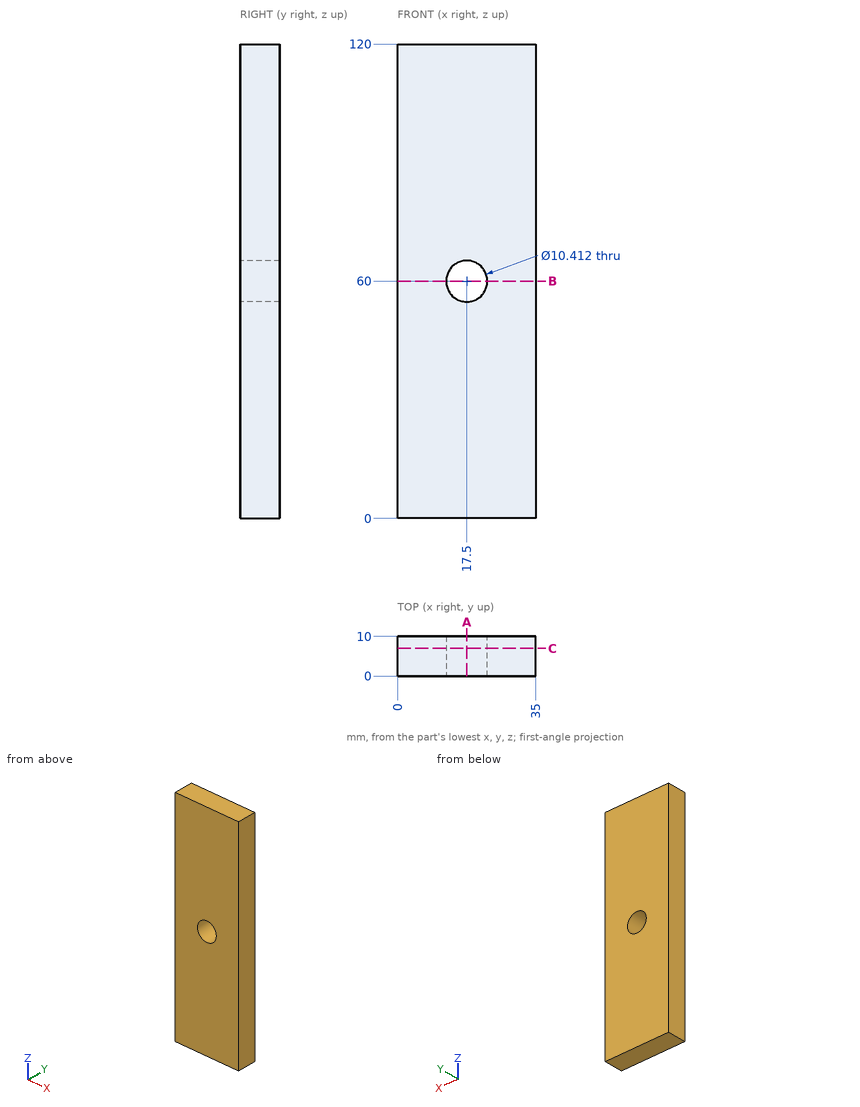
Here's the drawing with two shaded views (mm, measured from the low corner). I have some questions. Give positions to 0.01 mm unless a question says otherwise; leave off trailing zeros. Loops run counter-clockwise (first coordinate to the right, second up) from the corner with the lowest first, then second, coordinate; pieces in that order, holes last. Notation, with made-up numbers: M 0.25,2 L 37.25,2 A27 ccw 37.25,29 Z; hole C 89,24 d3. An arc over 180 degrees is marked long. Use one line per item in the form item = value. Start each with the question number.
Q1. I need wall thicknesses on line 1 along Z through (x, y) = (17.5, 4) (1 decimal); line 2 along X through (y, z) = (8.5, 60.5); line 3 along Z through (x, y) = (16.5, 5.5). Which ranges of each line are inside material? Lowest first, please.
Q2. If we section it at A-A (x = 17.5): Write out the boundary of the cut face in (y, z) (1 decimal), then the cut area to 3 significant figures.
Q3. If we section it at C-C (y = 7): Write out the boundary of the cut face in (x, z) (1 decimal), then the cut area to 4 significant figures.
Q4. If we section it at B-B (z = 60): Write out the boundary of the cut face in (x, y) (1 decimal).
Taken from the geometry:
q1.line_1 = 0 to 54.8, 65.2 to 120
q1.line_2 = 0 to 12.32, 22.68 to 35
q1.line_3 = 0 to 54.89, 65.11 to 120
q2.outline = M 0,0 L 10,0 L 10,54.8 L 0,54.8 Z; M 0,65.2 L 10,65.2 L 10,120 L 0,120 Z
q2.area = 1,100 mm^2
q3.outline = M 0,0 L 35,0 L 35,120 L 0,120 Z; hole C 17.5,60 d10.4
q3.area = 4,115 mm^2
q4.outline = M 0,0 L 12.3,0 L 12.3,10 L 0,10 Z; M 22.7,0 L 35,0 L 35,10 L 22.7,10 Z
